Geometry: final body of the model. Coordinates: model frame, mm. A direction names the side the tool comes from. Round coordinates to 2 decimals unless told otherwise and drop trailing zeros. Order: outer loops, then holes, each group sorted by start corner. A loop starts at its lowest first (then second) coordinate and runs counter-clockwise, first axis right, second up. Notation, with made-up numbers: (-25.75, -20.5) -> (27.25, -20.5) arc R32 ccw to (27.25, 18.5) -> close; hole circle Ø5 at (72, 18.25). An arc over 180 degrees is marked (long way). Put each result on its own line as item: value.
```python
from build123d import *

# Parameters (mm, degrees)
DODANIE_WYCI_GNI_CIE1_DEPTH = 40
SZKIC2_W                    = 30
SZKIC2_H                    = 2.5
WYTNIJ_WYCI_GNI_CIE1_DEPTH  = 164.095064303
EBRO3_START                 = -5
EBRO3_DEPTH                 = 5
SZKIC4_R                    = 4.5
WYTNIJ_WYCI_GNI_CIE2_DEPTH  = 10
SFAZOWANIE1_SIZE            = 0.5
WYTNIJ_WYCI_GNI_CIE3_DEPTH  = 10
DODANIE_WYCI_GNI_CIE2_START = 0.5
SZKIC6_R                    = 6
SZKIC6_R_2                  = 5.5
DODANIE_WYCI_GNI_CIE2_DEPTH = 0.5


# Read off the part's stored shape, not the designer's step: Żebro3
with BuildPart() as part:
    # Szkic1 → Dodanie-wyciągnięcie1 (new body)
    with BuildSketch(Plane(origin=(0, 0, 0), x_dir=(0, 0, -1), z_dir=(1, 0, 0))):
        Polygon((0, 0), (0, 50), (150, 50), (150, 45), (5, 45), (5, 0), align=None)
    extrude(amount=DODANIE_WYCI_GNI_CIE1_DEPTH)

    # Szkic2 → Wytnij-wyciągnięcie1 (cut, through all)
    with BuildSketch(Plane(origin=(0, 50, 0), x_dir=(1, 0, 0), z_dir=(0, 1, 0))):
        with Locations((20, 1.25)):
            Rectangle(SZKIC2_W, SZKIC2_H)
    extrude(amount=-WYTNIJ_WYCI_GNI_CIE1_DEPTH, mode=Mode.SUBTRACT)

    # Żebro3 outline → Żebro3 (add)
    with BuildSketch(Plane(origin=(40, 0, 0), x_dir=(0, 0, -1), z_dir=(1, 0, 0)).offset(EBRO3_START)):
        Polygon((5, 30), (30, 45), (5, 45), align=None)
    ebro3 = extrude(amount=EBRO3_DEPTH)

    # Lustro1: Żebro3 across plane
    add(ebro3.mirror(Plane(origin=(20, 0, 0), x_dir=(0, 0, 1), z_dir=(1, 0, 0))))

    # Szkic4 → Wytnij-wyciągnięcie2 (cut)
    with BuildSketch(Plane(origin=(0, 0, -5), x_dir=(-1, 0, 0), z_dir=(0, 0, -1))):
        with Locations((-20, 20)):
            Circle(SZKIC4_R)
    extrude(amount=-WYTNIJ_WYCI_GNI_CIE2_DEPTH, mode=Mode.SUBTRACT)

    # Sfazowanie1
    sfazowanie1_edges = [part.edges().sort_by_distance(p)[0] for p in [
        (24.5, 20, -2.5),
        (24.5, 20, -5),
    ]]
    chamfer(sfazowanie1_edges, length=SFAZOWANIE1_SIZE)

    # Szkic5 → Wytnij-wyciągnięcie3 (cut)
    with BuildSketch(Plane(origin=(0, 50, 0), x_dir=(1, 0, 0), z_dir=(0, 1, 0))):
        with BuildLine():
            ThreePointArc((20, 129.597336258), (14.5, 124.097336258), (20, 118.597336258))
            Line((20, 118.597336258), (20, 129.597336258))
        make_face()
        with BuildLine():
            Line((20, 129.597336258), (20, 118.597336258))
            ThreePointArc((20, 118.597336258), (23.889087297, 120.208248962), (25.5, 124.097336258))
            ThreePointArc((25.5, 124.097336258), (23.889087297, 127.986423555), (20, 129.597336258))
        make_face()
    extrude(amount=-WYTNIJ_WYCI_GNI_CIE3_DEPTH, mode=Mode.SUBTRACT)

    # Szkic6 → Dodanie-wyciągnięcie2 (add)
    with BuildSketch(Plane(origin=(0, 50, 0), x_dir=(1, 0, 0), z_dir=(0, 1, 0)).offset(DODANIE_WYCI_GNI_CIE2_START)):
        with Locations(Location((20, 124.097336258, 0), (0, 0, 270))):
            Circle(SZKIC6_R)
        with Locations(Location((20, 124.097336258, 0), (0, 0, 270))):
            Circle(SZKIC6_R_2, mode=Mode.SUBTRACT)
    extrude(amount=-DODANIE_WYCI_GNI_CIE2_DEPTH)


solid = part.part
```
1. Cut plane A-A on y = 20. Return loops of the section in (x, z).
Ans:
outline: (0, -5) -> (15, -5) -> (15.5, -4.5) -> (15.5, -3) -> (15, -2.5) -> (5, -2.5) -> (5, 0) -> (0, 0) -> close; (24.5, -4.5) -> (25, -5) -> (40, -5) -> (40, 0) -> (35, 0) -> (35, -2.5) -> (25, -2.5) -> (24.5, -3) -> close
2. Cut plane D-D on x = 28.5. Return loops of the section in (y, z), and give its area (3 significant figures).
Ans:
outline: (0, -5) -> (45, -5) -> (45, -150) -> (50, -150) -> (50, -2.5) -> (0, -2.5) -> close
area: 850 mm²
3. Set-up query: faces 1 (the face through (5, 25, -1)), 2 (the face through (35, 39, -15)), 3 (the face through (37.47, 37.4, -17.33)). Return all of +Z, -Z, +X, -X, +Y, -Y with unobstructed straight access to the full face (end or side cutting, diameter ignored); none if empty.
Ans:
face 1: +Z, +Y, -Y
face 2: -Z, -Y
face 3: -Z, +X, -X, -Y
4. Cut plane B-B on y = 46.5. Return loops of the section in (x, z).
Ans:
outline: (0, -150) -> (40, -150) -> (40, 0) -> (35, 0) -> (35, -2.5) -> (5, -2.5) -> (5, 0) -> (0, 0) -> close; hole circle Ø11 at (20, -124.1)
5. Contact query for flat-ended pins moving along their axis: P1, Ø8, axis at x = 27.5, y = 22, coming from the -Z side; P2, Ø4, axis at x = 19, z = -79.5, coming from the -Y side. Output: stop coordinate, or through.
Ans:
P1: z = -5
P2: y = 45
6. Draft query along X for faces 4 (the face through (20, 48, -150)), 5 (the face through (21.802, 50.254, -118.374)), 6 (the face through (19.8, 25.4, -2.5)). Return one class per face: +X half, -X half, draft (parallel to the pull), parting line (faces both ways), or undercut.
Ans:
face 4: draft
face 5: parting line
face 6: undercut
7. Material intervals for probe 1 along Z at (x, y) = (20, 46); probe 2 along Y at (x, z) = (20, -3.6); probe 3 along Z at (x, y) = (12, 24), sorted ascending.
Ans:
probe 1: -150 to -129.6, -118.6 to -2.5
probe 2: 0 to 15.5, 24.5 to 50
probe 3: -5 to -2.5
8. Cut plane C-C on z = -12. Return loops of the section in (x, y), and give its area (3 significant figures).
Ans:
outline: (0, 34.2) -> (5, 34.2) -> (5, 45) -> (35, 45) -> (35, 34.2) -> (40, 34.2) -> (40, 50) -> (0, 50) -> close
area: 308 mm²
